Autodesk Inventor part; units mm, degrees
ref_plane "YZ Plane" through (0, 0, 0) normal (1, 0, 0) x (0, 1, 0)
ref_plane "XZ Plane" through (0, 0, 0) normal (0, 1, 0) x (-1, 0, 0)
ref_plane "XY Plane" through (0, 0, 0) normal (0, 0, 1) x (1, 0, 0)
sketch "Clock Front Face Outline" plane through (0, 0, 0) normal (0, 0, 1) x (1, 0, 0)
  arc A0 (261.5609, 58.5131) -> (100.3256, 67.9894) centre (0, -3015.4231) ccw
  arc A1 (-100.3256, 67.9894) -> (-261.5609, 58.5131) centre (0, -3015.4231) ccw
  line L0 (-159.5034, -75) -> (159.5034, -75)
  arc A2 (-263.2612, -68.2167) -> (-160.4975, -74.9753) centre (0, 3150) ccw
  arc A3 (160.4975, -74.9753) -> (263.2612, -68.2167) centre (0, 3150) ccw
  arc A4 (300, 16.6643) -> (261.5609, 58.5131) centre (258, 16.6643) ccw
  arc A5 (263.2612, -68.2167) -> (300, -28.3498) centre (260, -28.3498) ccw
  arc A6 (-300, -28.3498) -> (-263.2612, -68.2167) centre (-260, -28.3498) ccw
  arc A7 (-261.5609, 58.5131) -> (-300, 16.6643) centre (-258, 16.6643) ccw
  arc A8 (-99.6752, 68) -> (-100.3256, 67.9894) centre (-99.6752, 48) ccw
  arc A9 (100.3256, 67.9894) -> (99.6752, 68) centre (99.6752, 48) ccw
  arc A10 (159.5034, -75) -> (160.4975, -74.9753) centre (159.5034, -55) ccw
  arc A11 (-160.4975, -74.9753) -> (-159.5034, -75) centre (-159.5034, -55) ccw
  line L1 (-99.6752, 68) -> (99.6752, 68)
  line L2 (300, 16.6643) -> (300, -28.3498)
  line L3 (-300, -28.3498) -> (-300, 16.6643)
  point P0 (0, -2.2582)
  point P1 (-300, 55)
  point P2 (300, 55)
  point P3 (-300, -65)
  point P4 (300, -65)
  point P5 (-160, -75)
  point P6 (160, -75)
  point P7 (-100, 68)
  point P8 (100, 68)
  dimension "d0" = 600
  dimension "d1" = 120
  dimension "d2" = 120
  dimension "d3" = 140
  dimension "d4" = 140
  dimension "d5" = 200
  dimension "d6" = 200
  dimension "d7" = 200
  dimension "d8" = 320
  dimension "d9" = 143
  dimension "d10" = 10
  dimension "d11" = 10
  dimension "d12" = 13
  dimension "d13" = 13
  dimension "d14" = 42
  dimension "d15" = 40
  dimension "d16" = 40
  dimension "d17" = 42
  dimension "d18" = 20
sketch "Sketch1" plane through (0, 0, 0) normal (0, 0, 1) x (1, 0, 0)
  arc A0 (261.5609, 58.5131) -> (100.3256, 67.9894) centre (0, -3015.4231) ccw
  arc A1 (-100.3256, 67.9894) -> (-261.5609, 58.5131) centre (0, -3015.4231) ccw
  line L0 (-159.5034, -75) -> (159.5034, -75)
  arc A2 (-263.2612, -68.2167) -> (-160.4975, -74.9753) centre (0, 3150) ccw
  arc A3 (160.4975, -74.9753) -> (263.2612, -68.2167) centre (0, 3150) ccw
  arc A4 (300, 16.6643) -> (261.5609, 58.5131) centre (258, 16.6643) ccw
  arc A5 (263.2612, -68.2167) -> (300, -28.3498) centre (260, -28.3498) ccw
  arc A6 (-300, -28.3498) -> (-263.2612, -68.2167) centre (-260, -28.3498) ccw
  arc A7 (-261.5609, 58.5131) -> (-300, 16.6643) centre (-258, 16.6643) ccw
  arc A8 (-99.6752, 68) -> (-100.3256, 67.9894) centre (-99.6752, 48) ccw
  arc A9 (100.3256, 67.9894) -> (99.6752, 68) centre (99.6752, 48) ccw
  arc A10 (159.5034, -75) -> (160.4975, -74.9753) centre (159.5034, -55) ccw
  arc A11 (-160.4975, -74.9753) -> (-159.5034, -75) centre (-159.5034, -55) ccw
  line L1 (-99.6752, 68) -> (99.6752, 68)
  line L2 (300, 16.6643) -> (300, -28.3498)
  line L3 (-300, -28.3498) -> (-300, 16.6643)
  point P0 (0, 0)
  point P1 (0, 0)
  dimension "d19" = 300
  dimension "d20" = 75
extrude "Extrusion1" add sketch "Sketch1" along normal blind 0.5
properties part number "7 Segment Clock Blanking Plate" material "PMMA PlasticBlack"
Model file for the job. Use its own axes, mm. Give positions to 0.01 mm unless a question says otherwise; leave off trailing zeros. Write each loop counter-clockwise with the first axis right and the second up, starting at its lowest first coordinate (ties: lowest second). Pieces come first, ordered by that corner, then holes. Notation, with made-up numbers: M 24,17 L 69,17 A28 ccw 69,56 Z; hole C 5.5,-26.75 d3. An arc over 180 degrees is marked long. One line per item, written item: value. Start each with the question number.
Q1. Drop a flat-ended pin along its axis: pin 1 Ø4 at (x, y) = (-47.5, -50.5) entering from -Z. Give the stop position or say it passes through.
Q2. Saw through at B-B, the plane x = -166.5. Write the cut outline in (y, z), plus the area to 3 significant figures.
Q3. Saw through at C-C, the plane y = 47. Write the cut outline in (x, z).
Q4. Probe probe 1 along X at (y, z) = (-47.5, 0.2); probe 2 along X at (y, z) = (29, 0.1); probe 3 along Y at (x, z) = (142, 0.4). List the from-to ranges inside material, lowest first. Write a range as [from, to].
Q5. Saw through at A-A, the plane z = 0.35. Write the cut outline in (x, y), plus the area to 3 significant figures.
Output values:
1. pin 1: stops at z = 0
2. outline: M -74.67,0 L 65.12,0 L 65.12,0.5 L -74.67,0.5 Z
2. area: 69.9 mm²
3. outline: M -287.05,0 L 287.05,0 L 287.05,0.5 L -287.05,0.5 Z
4. probe 1: x = [-295.12, 295.12]
4. probe 2: x = [-298.15, 298.15]
4. probe 3: y = [-75, 66.35]
5. outline: M -300,-28.35 A40 ccw -263.26,-68.22 A3228.93 ccw -160.5,-74.98 A19.97 ccw -159.5,-75 L 159.5,-75 A20.03 ccw 160.5,-74.98 A3229 ccw 263.26,-68.22 A40 ccw 300,-28.35 L 300,16.66 A42 ccw 261.56,58.51 A3085.05 ccw 100.33,67.99 A20.08 ccw 99.68,68 L -99.68,68 A19.92 ccw -100.33,67.99 A3085.04 ccw -261.56,58.51 A42 ccw -300,16.66 Z
5. area: 81,200 mm²
